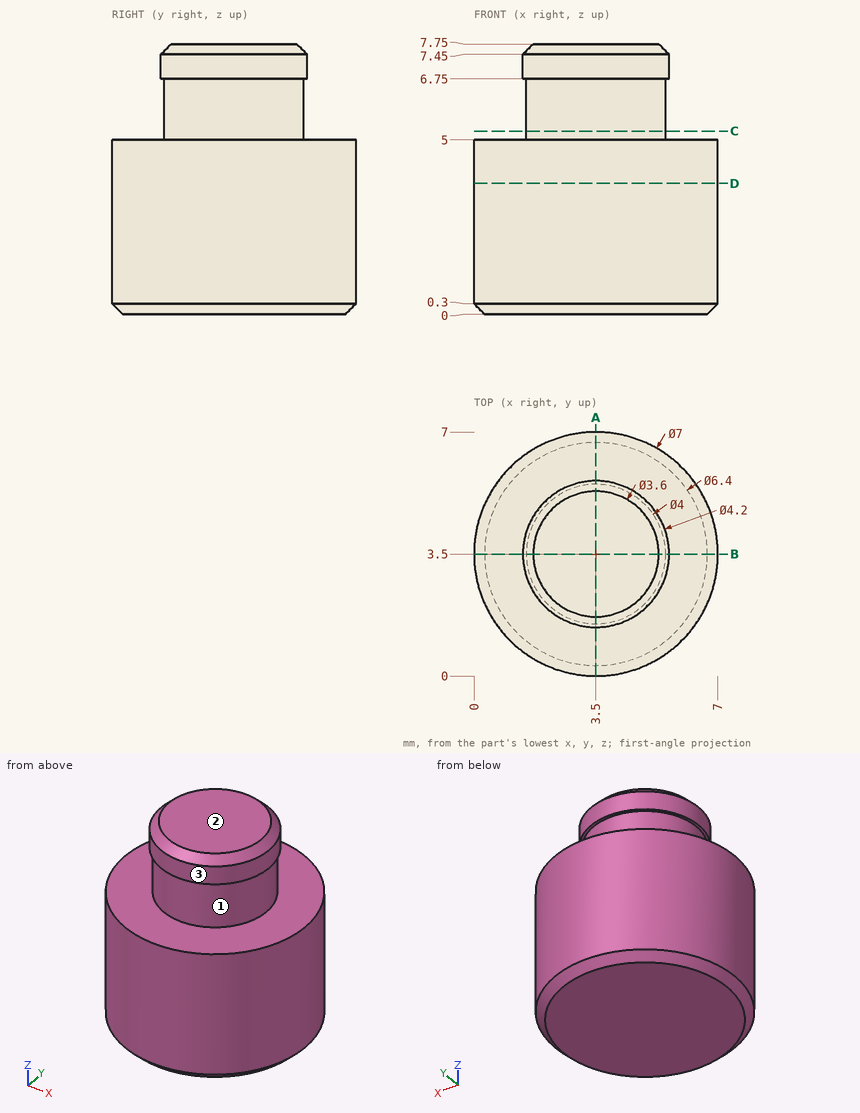
Verification items for this drawing (mm, ordinates from the low corner). Give positions to 0.01 mm unless a question says otherwise; leave off trailing zeros. Write each loop counter-clockwise with the first axis right and the second up, starting at its lowest first coordinate (ties: lowest second). Pieces come first, ordered by that corner, then holes. Notation, with made-up numbers: (36.25, -23.75) - (43.25, -23.75) arc R22 cw to (43.25, -12.75) - close; hole circle Ø7 at (80, -1). An arc over 180 degrees is marked (long way). Answer as a JSON object with one key per item and string values. Group by question number.
1) Sectioned sample at A-A (x = 3.5). Record the cut outline in (y, z).
2) Release check for a two-part mould opening along Z. For the marked faces 1, 2 and 3 record: pulls with the +Z half, pulls with the -Z half, needs draft (parallel to the pull), parting line crosses it, or undercut.
3) Sectioned sample at D-D (z = 3.75). Record the cut outline in (x, y), then the cut area to 3 significant figures.
4) Thickness scan on probe 1 along Z at (x, y) = (3.75, 1); probe 2 along X at (y, z) = (6.5, 1.75); probe 3 along Y at (x, z) = (5.75, 1.25). Record the ranges inside material, lowest first. Write a range as from..to.
5) Sectioned sample at C-C (z = 5.25). Record the cut outline in (x, y), then the cut area to 3 significant figures.
6) Depth check by flat-ended pin: P1, Ø1, axis at y = 3, z = 7, coming from the +X side; P2, Ø1.5, axis at y = 4.5, z = 6, coming from the +X side; P3, Ø2, axis at x = 2.5, z = 7, coming from the +Y side. Enter the tip coordinate at first touch or a pass-through.
Geometry results:
{
 "1": {"outline": "(0, 0.3) - (0.3, 0) - (6.7, 0) - (7, 0.3) - (7, 5) - (5.5, 5) - (5.5, 6.75) - (5.6, 6.75) - (5.6, 7.45) - (5.3, 7.75) - (1.7, 7.75) - (1.4, 7.45) - (1.4, 6.75) - (1.5, 6.75) - (1.5, 5) - (0, 5) - close"},
 "2": {"face 1": "undercut", "face 2": "pulls with the +Z half", "face 3": "needs draft"},
 "3": {"outline": "circle Ø7 at (3.5, 3.5)", "area": "38.5 mm^2"},
 "4": {"probe 1": "z = 0..5", "probe 2": "x = 1.7..5.3", "probe 3": "y = 0.82..6.18"},
 "5": {"outline": "circle Ø4 at (3.5, 3.5)", "area": "12.6 mm^2"},
 "6": {"P1": "stops at x = 5.6", "P2": "stops at x = 5.48", "P3": "stops at y = 5.6"}
}
